Autodesk Inventor part; units mm, degrees
ref_plane "YZ Plane" through (0, 0, 0) normal (1, 0, 0) x (0, 1, 0)
ref_plane "XZ Plane" through (0, 0, 0) normal (0, 1, 0) x (-1, 0, 0)
ref_plane "XY Plane" through (0, 0, 0) normal (0, 0, 1) x (1, 0, 0)
sketch "Sketch1" plane through (0, 0, 0) normal (1, 0, 0) x (0, 1, 0)
  circle A0 centre (52.468, 74.8832) radius 4
  circle A1 centre (81.968, 24.8832) radius 4
  circle A2 centre (29.468, 45.8832) radius 12
  circle A3 centre (13.968, 61.3832) radius 1.5
  circle A4 centre (43.968, 61.3832) radius 1.5
  circle A5 centre (43.968, 31.3832) radius 1.5
  circle A6 centre (13.968, 31.3832) radius 1.5
  arc A7 (61.2976, 79.5777) -> (47.3885, 83.497) centre (52.468, 74.8832) ccw
  arc A8 (81.968, 14.8832) -> (90.2193, 30.5327) centre (81.968, 24.8832) ccw
  line L0 (60.8493, 80.3379) -> (90.9051, 29.3697)
  line L1 (47.3885, 83.497) -> (7.3003, 68.8293)
  line L2 (3.968, 61.3832) -> (3.968, 67.6101)
  line L3 (7.3003, 68.8293) -> (3.968, 67.6101)
  line L4 (3.968, 61.3832) -> (3.968, 14.8832)
  line L5 (81.968, 14.8832) -> (3.968, 14.8832)
  point P0 (0, 0)
extrude "Extrusion1" add sketch "Sketch1" along normal blind 10 contours L0 A8 L5 L4 L2 L3 L1 A7
properties part number "Y_MotorMount" material "Birch"
Source: CAD feature listing. Evaluate the final solid. Frame: model axes, mm. Give positions to 0.01 mm unless a question says otherwise; leave off trailing zeros. Order: outer loops, then holes, each group sorted by start corner. A loop starts at its lowest first (then second) coordinate and runs counter-clockwise, first axis right, second up. Notation, with made-up numbers: (-5.5, 34) -> (17.5, 34) arc R24 ccw to (17.5, 51) -> close; hole circle Ø7 at (-37.5, 45.25). An arc over 180 degrees is marked (long way). Use a Markdown table: item, result.
Q1. Section C-C (x = 2). Return the cut outline in (y, z).
A:
| item | result |
|---|---|
| outline | (3.97, 14.88) -> (81.97, 14.88) arc R10 ccw to (90.91, 29.37) -> (60.85, 80.34) arc R10 ccw to (47.39, 83.5) -> (7.3, 68.83) -> (3.97, 67.61) -> close; hole circle Ø3 at (13.97, 31.38); hole circle Ø3 at (13.97, 61.38); hole circle Ø24 at (29.47, 45.88); hole circle Ø3 at (43.97, 31.38); hole circle Ø3 at (43.97, 61.38); hole circle Ø8 at (52.47, 74.88); hole circle Ø8 at (81.97, 24.88) |
Q2. Section D-D (y = 30.5). Return the cut outline in (x, z).
A:
| item | result |
|---|---|
| outline | (0, 14.88) -> (10, 14.88) -> (10, 33.93) -> (0, 33.93) -> close; (0, 57.84) -> (10, 57.84) -> (10, 77.32) -> (0, 77.32) -> close |
Q3. Section A-A (z = 47.5). Return the cut outline in (x, y), and give its area (3 significant figures).
A:
| item | result |
|---|---|
| outline | (0, 3.97) -> (10, 3.97) -> (10, 17.58) -> (0, 17.58) -> close; (0, 41.36) -> (10, 41.36) -> (10, 80.21) -> (0, 80.21) -> close |
| area | 525 mm^2 |
Q4. Material intervals for line 1 (Z direction, x = 5.5, y = 14.5); line 2 (Y direction, x = 9.5, z = 51.5); line 3 (Z direction, x = 7.75, y = 26.5), sorted ascending. Write a range as [from, to].
A:
| item | result |
|---|---|
| line 1 | [14.88, 29.98], [32.79, 59.98], [62.79, 71.46] |
| line 2 | [3.97, 18.86], [40.07, 77.85] |
| line 3 | [14.88, 34.26], [57.51, 75.85] |
Q5. Pull-direction query (Z, two-part tool) for faces 1 (the face through (4.93, 90.55, 19.75)), 2 (the face through (4.93, 14.66, 62.714)), 3 (the face through (4.93, 54.649, 84.643)); classes: +Z half, -Z half, draft (parallel to the pull), parting line (faces both ways), or undercut.
A:
| item | result |
|---|---|
| face 1 | parting line |
| face 2 | undercut |
| face 3 | +Z half |
Q6. Section B-B (y = 14). Return the cut outline in (x, z).
A:
| item | result |
|---|---|
| outline | (0, 14.88) -> (10, 14.88) -> (10, 29.88) -> (0, 29.88) -> close; (0, 32.88) -> (10, 32.88) -> (10, 59.88) -> (0, 59.88) -> close; (0, 62.88) -> (10, 62.88) -> (10, 71.28) -> (0, 71.28) -> close |
Q7. First-contact query: P1, Ø3.5, axis at y = 43.97, z = 61.38, coming from the -X side; P2, Ø5, axis at x = 7.5, y = 77.5, coming from the +Z side. Flat tips, straight axial feed; report the tip coordinate or a pass-through.
A:
| item | result |
|---|---|
| P1 | x = 0 |
| P2 | z = 56.34 |
